Design review of the part built by this model. Coordinates are the model's own, in mm. Coordinates: 2 decimals unless noted, no trailing zeros. Write each loop counter-clockwise with the first axis right and the second up, starting at its lowest first coordinate (ties: lowest second). Pieces come first, ordered by that corner, then holes.
```python
from build123d import *

# Parameters (mm, degrees)
F0_R     = 2
F1_DEPTH = 1


with BuildPart() as f1:
    # F0 (on Front) → F1 (new body)
    with BuildSketch(Plane.XZ):
        with BuildLine():
            ThreePointArc((95.666444, 72.442608), (105.390764, 57.382809), (112.763114, 41.042417))
            ThreePointArc((112.763114, 41.042417), (122.589579, 36.460262), (127.171735, 46.286726))
            Line((127.171735, 46.286726), (129.05112, 46.970766))
            ThreePointArc((129.05112, 46.970766), (138.877584, 42.388611), (143.45974, 52.215075))
            Line((143.45974, 52.215075), (145.339125, 52.899116))
            ThreePointArc((145.339125, 52.899116), (155.16559, 48.31696), (159.747746, 58.143424))
            ThreePointArc((159.747746, 58.143424), (-170, 0), (159.747746, -58.143424))
            ThreePointArc((159.747746, -58.143424), (155.16559, -48.31696), (145.339125, -52.899116))
            Line((145.339125, -52.899116), (143.45974, -52.215075))
            ThreePointArc((143.45974, -52.215075), (138.877584, -42.388611), (129.05112, -46.970766))
            Line((129.05112, -46.970766), (127.171735, -46.286726))
            ThreePointArc((127.171735, -46.286726), (122.589579, -36.460262), (112.763114, -41.042417))
            ThreePointArc((112.763114, -41.042417), (105.390764, -57.382809), (95.666444, -72.442608))
            ThreePointArc((95.666444, -72.442608), (95.761119, -73.144091), (95.05944, -73.237305))
            Line((95.05944, -73.237305), (78.972507, -59.738765))
            ThreePointArc((78.972507, -59.738765), (76.052734, -58.818164), (73.337179, -60.231792))
            Line((73.337179, -60.231792), (72.051604, -61.763881))
            ThreePointArc((72.051604, -61.763881), (71.131003, -64.683655), (72.544631, -67.399209))
            Line((72.544631, -67.399209), (88.631564, -80.897749))
            ThreePointArc((88.631564, -80.897749), (88.661612, -81.604954), (87.954346, -81.633529))
            ThreePointArc((87.954346, -81.633529), (31.058285, -115.911099), (-35.353934, -114.673883))
            ThreePointArc((-35.353934, -114.673883), (-35.980731, -115.002769), (-36.308312, -114.375288))
            Line((-36.308312, -114.375288), (-29.125889, -94.641743))
            ThreePointArc((-29.125889, -94.641743), (-29.259428, -91.583189), (-31.516578, -89.514892))
            Line((-31.516578, -89.514892), (-33.395964, -88.830852))
            ThreePointArc((-33.395964, -88.830852), (-36.454517, -88.964391), (-38.522815, -91.221542))
            Line((-38.522815, -91.221542), (-45.705238, -110.955087))
            ThreePointArc((-45.705238, -110.955087), (-46.359516, -111.225201), (-46.628266, -110.570361))
            ThreePointArc((-46.628266, -110.570361), (-98.298245, -68.829172), (-119.849959, -5.998947))
            ThreePointArc((-119.849959, -5.998947), (-120.373389, -5.522436), (-119.895788, -5))
            Line((-119.895788, -5), (-98.895788, -5))
            ThreePointArc((-98.895788, -5), (-96.067361, -3.828427), (-94.895788, -1))
            Line((-94.895788, -1), (-94.895788, 1))
            ThreePointArc((-94.895788, 1), (-96.067361, 3.828427), (-98.895788, 5))
            Line((-98.895788, 5), (-119.895788, 5))
            ThreePointArc((-119.895788, 5), (-120.373389, 5.522436), (-119.849959, 5.998947))
            ThreePointArc((-119.849959, 5.998947), (-98.298245, 68.829172), (-46.628266, 110.570361))
            ThreePointArc((-46.628266, 110.570361), (-46.359516, 111.225201), (-45.705238, 110.955087))
            Line((-45.705238, 110.955087), (-38.522815, 91.221542))
            ThreePointArc((-38.522815, 91.221542), (-36.454517, 88.964391), (-33.395964, 88.830852))
            Line((-33.395964, 88.830852), (-31.516578, 89.514892))
            ThreePointArc((-31.516578, 89.514892), (-29.259428, 91.583189), (-29.125889, 94.641743))
            Line((-29.125889, 94.641743), (-36.308312, 114.375288))
            ThreePointArc((-36.308312, 114.375288), (-35.980731, 115.002769), (-35.353934, 114.673883))
            ThreePointArc((-35.353934, 114.673883), (31.058285, 115.911099), (87.954346, 81.633529))
            ThreePointArc((87.954346, 81.633529), (88.661612, 81.604954), (88.631564, 80.897749))
            Line((88.631564, 80.897749), (72.544631, 67.399209))
            ThreePointArc((72.544631, 67.399209), (71.131003, 64.683655), (72.051604, 61.763881))
            Line((72.051604, 61.763881), (73.337179, 60.231792))
            ThreePointArc((73.337179, 60.231792), (76.052734, 58.818164), (78.972507, 59.738765))
            Line((78.972507, 59.738765), (95.05944, 73.237305))
            ThreePointArc((95.05944, 73.237305), (95.761119, 73.144091), (95.666444, 72.442608))
        make_face()
        with Locations((119.967425, -43.664572)):
            Circle(F0_R, mode=Mode.SUBTRACT)
        with Locations((136.25543, -49.592921)):
            Circle(F0_R, mode=Mode.SUBTRACT)
        with Locations((152.543435, -55.52127)):
            Circle(F0_R, mode=Mode.SUBTRACT)
        with Locations((119.967425, 43.664572)):
            Circle(F0_R, mode=Mode.SUBTRACT)
        with Locations((136.25543, 49.592921)):
            Circle(F0_R, mode=Mode.SUBTRACT)
        with Locations((152.543435, 55.52127)):
            Circle(F0_R, mode=Mode.SUBTRACT)
    extrude(amount=F1_DEPTH)


solid = f1.part
```
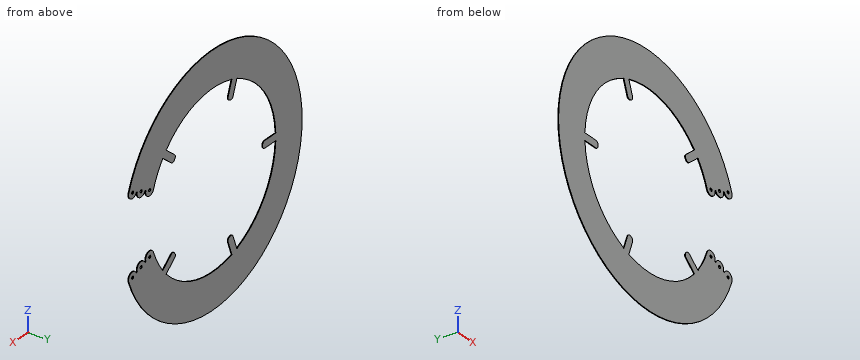
(1) Consider section C-C (x = -70). Give the boundary of the cut face in (y, z), plus the area to 3 significant figures.
(2) Wall thickness on line 1 (X direction, y = -0.4, z = -93); line 2 (X direction, y = -0.65, z = -99); line 3 (Z direction, x = 3, y = -0.1): over which ranges is each line inside the solid? List them lowest first.
(3) Consider section D-D (y = -0.3). State how many separate pieces and enclosed holes the cut face has, plus the area to 3 significant figures.
(4) Consider section A-A (x = 0). Give the boundary of the cut face in (y, z), plus the area to 3 significant figures.
(5) Insertion check: pin 1 Ø3 at (x, z) = (152.54, 55.52) entering from +Y; pin 2 Ø0.5 at (y, z) = (-0.5, 0.5) entering from +X; pin 3 Ø0.5 at (x, y) = (-110.5, -0.5) entering from +Z. Each pin has a flat end and moves straight along its axis. Give the tip position at first contact, or say it passes through.
(6) Consider section B-B (z = -101). Give the boundary of the cut face in (x, y).
Results:
1. outline: (-1, -154.92) - (0, -154.92) - (0, -97.47) - (-1, -97.47) - close; (-1, 97.47) - (0, 97.47) - (0, 154.92) - (-1, 154.92) - close
1. area: 115 mm2
2. line 1: x = -142.31 to -75.84, -39.17 to -28.89, 75.84 to 142.31
2. line 2: x = -138.2 to -67.82, -41.35 to -30.71, 67.82 to 138.2
2. line 3: z = -169.97 to -119.96, 119.96 to 169.97
3. separate pieces: 1
3. enclosed holes: 6
3. area: 42,200 mm2
4. outline: (-1, -170) - (0, -170) - (0, -120) - (-1, -120) - close; (-1, 120) - (0, 120) - (0, 170) - (-1, 170) - close
4. area: 100 mm2
5. pin 1: passes through
5. pin 2: stops at x = -94.9
5. pin 3: stops at z = 129.4
6. outline: (-136.74, -1) - (-64.8, -1) - (-64.8, 0) - (-136.74, 0) - close; (-42.08, -1) - (-31.44, -1) - (-31.44, 0) - (-42.08, 0) - close; (64.8, -1) - (136.74, -1) - (136.74, 0) - (64.8, 0) - close
